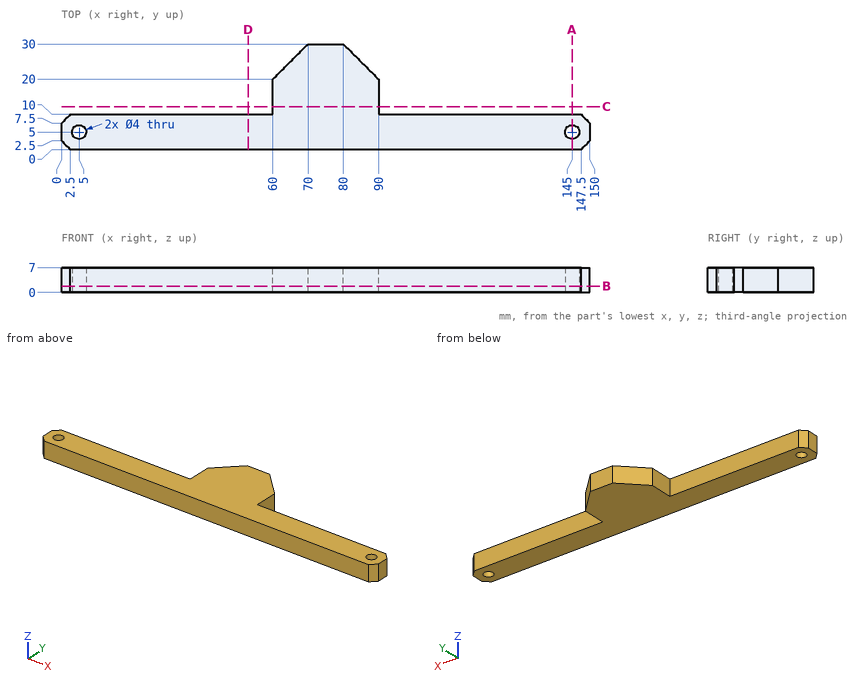
Drawing for the job (mm, zero at the part's lowest x, y, z). Round coordinates to 2 decimals unless told otherwise and drop trailing zeros. Order: outer loops, then holes, each group sorted by start corner. A loop starts at its lowest first (then second) coordinate and runs counter-clockwise, first axis right, second up. Notation, with made-up numbers: (55, -16.5) -> (111, -16.5) arc R11 cw to (111, 1.5) -> close; hole circle Ø5 at (-27, 83.25). An arc over 180 degrees is marked (long way). Write item = value, one per line. Start each with the question number.
(1) Cut at C-C, the plane y = 12.25. List the corners of the cut face in (x, z).
(2) Cut at D-D, the plane x = 53. List the corners of the cut face in (y, z).
(3) Cut at B-B, the plane z = 1.75. List the corners of the cut face in (x, y).
(4) Pin check, flat tips, straight feed: P1, Ø3, axis at x = 145, y = 5, coming from the -Z side; P2, Ø1.5, axis at x = 48, z = 6, coming from the +Y side; P3, Ø4, axis at y = 21, z = 2, coming from the +X side. Stop position of each tip, or through.
(5) Cut at A-A, the plane x = 145. List the corners of the cut face in (y, z), then the cut area to 3 significant figures.
(6) Probe line 1 (X direction, y = 5, z = 3.75); line 2 (Y direction, x = 5, z = 3.25); line 3 (Y direction, x = 16, z = 5.75). List the from-to ranges inside material, lowest first. Write a range as [from, to].
Model answer:
q1.outline = (60, 0) -> (90, 0) -> (90, 7) -> (60, 7) -> close
q2.outline = (0, 0) -> (10, 0) -> (10, 7) -> (0, 7) -> close
q3.outline = (0, 2.5) -> (2.5, 0) -> (147.5, 0) -> (150, 2.5) -> (150, 7.5) -> (147.5, 10) -> (90, 10) -> (90, 20) -> (80, 30) -> (70, 30) -> (60, 20) -> (60, 10) -> (2.5, 10) -> (0, 7.5) -> close; hole circle Ø4 at (5, 5); hole circle Ø4 at (145, 5)
q4.P1 = through
q4.P2 = 10
q4.P3 = 90
q5.outline = (0, 0) -> (3, 0) -> (3, 7) -> (0, 7) -> close; (7, 0) -> (10, 0) -> (10, 7) -> (7, 7) -> close
q5.area = 42.0 mm2
q6.line_1 = [0, 3], [7, 143], [147, 150]
q6.line_2 = [0, 3], [7, 10]
q6.line_3 = [0, 10]
